The model under review builds one solid part; all positions refer to its coordinate system, in mm. Round coordinates to 2 decimals unless told otherwise and drop trailing zeros. Write each loop counter-clockwise with the first axis right and the second up, starting at its lowest first coordinate (ties: lowest second). Pieces come first, ordered by that corner, then holes. Notation, with made-up numbers: (-12, 35) -> (32, 35) arc R17 ccw to (32, 46) -> close; hole circle Ø8 at (17.5, -23). An arc over 180 degrees is marked (long way). Return JSON: item names as keys, results as strings. Group by question number.
1. Take a section at D-D, the plane z = 0. Write out the cut boundary in (x, y), then the cut area to 3 significant figures.
2. Mouldability with a two-part tool opening along X and no side actions: class faces 1 (the cylindrical face through (-6.896, -1.232, 10.844)), 2 (the flat face through (-4, -1, 17.5)), 3 (the flat face through (-19.24, -1.232, 14.145)), 4 (the flat face through (15.402, -1, 1)) as pulls with the +X half, pulls with the -X half, needs draft (parallel to the pull), parting line crosses it, or undercut.
3. Take a section at A-A, the plane x = -10. Write out the cut boundary in (y, z).
4. Take a section at B-B, the plane y = -0.65. Write out the cut boundary in (x, z).
5. Clearance check with a flat-ended pin moving along its axis: P1, Ø4, axis at x = 7.9, z = 0, coming from the -Y side. State where the tip first meets the part, or that it passes through.
6. Take a section at C-C, the plane z = 4. Write out the cut boundary in (x, y).
7. For line 1 along X through (y, z) = (-2.1, 0.5); line 2 along X through (y, z) = (-1.2, 2.25); line 3 along X through (y, z) = (-0.1, 7.5), list the stretches that pass through material, from the lowest coordinate up. Write a range as from..to.
from build123d import *

# Parameters (mm, degrees)
F0_R     = 2.5
F0_R_2   = 6.25
F1_DEPTH = 2.5


with BuildPart() as f1:
    # F0 (on Front) → F1 (new body)
    with BuildSketch(Plane.XZ):
        Polygon((-14.030276, 17.5), (-24.598361, 10.694085), (-24.598361, -7.5), (15.401639, -7.5), (15.401639, 9.590163), (5.632331, 17.5), align=None)
        with Locations((-17.098361, 0)):
            Circle(F0_R, mode=Mode.SUBTRACT)
        with Locations((-6.081968, 4.647542)):
            Circle(F0_R_2, mode=Mode.SUBTRACT)
        with Locations((7.901639, 0)):
            Circle(F0_R, mode=Mode.SUBTRACT)
    extrude(amount=F1_DEPTH)


solid = f1.part
Output:
{
 "1": {"outline": "(-24.6, -2.5) -> (-19.6, -2.5) -> (-19.6, 0) -> (-24.6, 0) -> close; (-14.6, -2.5) -> (-10.26, -2.5) -> (-10.26, 0) -> (-14.6, 0) -> close; (-1.9, -2.5) -> (5.4, -2.5) -> (5.4, 0) -> (-1.9, 0) -> close; (10.4, -2.5) -> (15.4, -2.5) -> (15.4, 0) -> (10.4, 0) -> close", "area": "54.1 mm^2"},
 "2": {"face 1": "undercut", "face 2": "needs draft", "face 3": "pulls with the -X half", "face 4": "pulls with the +X half"},
 "3": {"outline": "(-2.5, -7.5) -> (0, -7.5) -> (0, -0.22) -> (-2.5, -0.22) -> close; (-2.5, 9.52) -> (0, 9.52) -> (0, 17.5) -> (-2.5, 17.5) -> close"},
 "4": {"outline": "(-24.6, -7.5) -> (15.4, -7.5) -> (15.4, 9.59) -> (5.63, 17.5) -> (-14.03, 17.5) -> (-24.6, 10.69) -> close; hole circle Ø5 at (-17.1, 0); hole circle Ø12.5 at (-6.08, 4.65); hole circle Ø5 at (7.9, 0)"},
 "5": {"P1": "passes through"},
 "6": {"outline": "(-24.6, -2.5) -> (-12.3, -2.5) -> (-12.3, 0) -> (-24.6, 0) -> close; (0.13, -2.5) -> (15.4, -2.5) -> (15.4, 0) -> (0.13, 0) -> close"},
 "7": {"line 1": "x = -24.6..-19.55, -14.65..-10.76, -1.41..5.45, 10.35..15.4", "line 2": "x = -24.6..-18.19, -16.01..-11.85, -0.31..6.81, 8.99..15.4", "line 3": "x = -24.6..-11.64, -0.52..15.4"}
}
